```python
from build123d import *

# Parameters (mm, degrees)
SKETCH2_W                       = 1
SKETCH2_H                       = 27.5
REVOLVE1_ANGLE                  = 130
SKETCH3_W                       = 1
SKETCH3_H                       = 27.5
BOSS_EXTRUDE1_DEPTH             = 7.5
SKETCH4_W                       = 1
SKETCH4_H                       = 27.5
BOSS_EXTRUDE2_DEPTH             = 7.5
M2_5_CLEARANCE_HOLE1_D          = 3.1
CIRPATTERN1_COUNT               = 2
CIRPATTERN1_ANGLE               = 65
CIRPATTERN1_THE_OTHER_WAY_COUNT = 2
CIRPATTERN1_THE_OTHER_WAY_ANGLE = 65


with BuildPart() as part:
    # Sketch2 → Revolve1 (revolve, symmetric)
    with BuildSketch(Plane(origin=(0, 0, 0), x_dir=(0, 0, -1), z_dir=(1, 0, 0))) as revolve1_sk:
        with Locations((-149.5, 0)):
            Rectangle(SKETCH2_W, SKETCH2_H)
    revolve(axis=Axis((0, -1000, 0), (0, 1, 0)), revolution_arc=REVOLVE1_ANGLE / 2)
    revolve(revolve1_sk.sketch, axis=Axis((0, -1000, 0), (0, -1, 0)), revolution_arc=REVOLVE1_ANGLE / 2)

    # Sketch3 → Boss-Extrude1 (add)
    with BuildSketch(Plane(origin=(0, 0, 0), x_dir=(-0.9063077870366509, 1.4496858692468702e-15, -0.4226182617406975), z_dir=(0.4226182617406975, 3.1088613791648487e-15, -0.9063077870366509))):
        with Locations((-149.5, 0)):
            Rectangle(SKETCH3_W, SKETCH3_H)
    extrude(amount=BOSS_EXTRUDE1_DEPTH)

    # Sketch4 → Boss-Extrude2 (add)
    with BuildSketch(Plane(origin=(0, 0, 0), x_dir=(-0.906307787036651, -1.4496858692468694e-15, 0.4226182617406973), z_dir=(-0.4226182617406973, 3.1088613791648455e-15, -0.906307787036651))):
        with Locations((149.5, 0)):
            Rectangle(SKETCH4_W, SKETCH4_H)
    extrude(amount=BOSS_EXTRUDE2_DEPTH)

    # M2.5 Clearance Hole1 (through all)
    with Locations(Plane(origin=(0, 0, 0), x_dir=(1, 0, 0), z_dir=(0, 0, -1))):
        with Locations((0, -10.575), (0, 10.575)):
            m2_5_clearance_hole1 = Hole(M2_5_CLEARANCE_HOLE1_D / 2)

    # CirPattern1: M2.5 Clearance Hole1 ×2 about axis
    cirpattern1_axis = Axis((0, -1000, 0), (0, 1, 0))
    for i in range(1, CIRPATTERN1_COUNT):
        add(m2_5_clearance_hole1.rotate(cirpattern1_axis, i * CIRPATTERN1_ANGLE / (CIRPATTERN1_COUNT - 1)), mode=Mode.SUBTRACT)

    # CirPattern1 the other way: M2.5 Clearance Hole1 ×2 about axis
    cirpattern1_the_other_way_axis = Axis((0, -1000, 0), (0, -1, 0))
    for i in range(1, CIRPATTERN1_THE_OTHER_WAY_COUNT):
        add(m2_5_clearance_hole1.rotate(cirpattern1_the_other_way_axis, i * CIRPATTERN1_THE_OTHER_WAY_ANGLE / (CIRPATTERN1_THE_OTHER_WAY_COUNT - 1)), mode=Mode.SUBTRACT)


solid = part.part
```
For this review, take the finished solid that the model builds, in its own axes (mm). A direction names the side the tool comes from. Give positions to 0.01 mm unless a question says otherwise; leave off trailing zeros. Loops run counter-clockwise (first coordinate to the right, second up) from the corner with the lowest first, then second, coordinate; pieces in that order, holes last. Notation, with made-up numbers: M 21,17.5 L 75,17.5 A34 ccw 75,55.5 Z; hole C -21,7 d5. An arc over 180 degrees is marked long. One line per item, written item: value. Start each with the question number.
Q1. Add section D-D (x = 108). Give the boundary of the cut face in (y, z).
Q2. Add section C-C (x = -25). Give the boundary of the cut face in (y, z), and give its area (3 significant figures).
Q3. For L1, parallel to X at y = -11.5, z = 132.5; L2, parallel to X at y = 0, z = 98.5; L3, parallel to Z at x = -2, y = -10.75, list the stretches that pass through material, from the lowest coordinate up.
Q4. Add section A-A (z = 93.5). Give the boundary of the cut face in (x, y), and give its area (3 significant figures).
Q5. Machinability: for faces 1 (the face through (2.38, 0.19, 149.98)), 2 (the face through (-136.6, -0.19, 59.62)), which of the approach directions +Z, -Z, +X, -X, +Y, -Y give a long, thin tool a straight path to every point of the face, cutting with its end or side? Answer none if there is none.
Q6. Clearance check with flat-ended pins moving along their axes: pin 1 Ø2 at (x, y) = (-44.5, -6.5) entering from +Z; pin 2 Ø5 at (x, y) = (-71.5, 1.5) entering from -Z; pin 3 Ø10 at (y, z) = (5.5, 126.5) entering from -X. State where each tip first meets the part, or that it passes through.
Q7. Add section B-B (y = 5.75). Give the boundary of the cut face in (x, z), and give its area (3 significant figures).
Q8. Draft analysis for pull direction X (two halves, no side actions). For faces 3 (the face through (137.51, -0.19, 60.04)), 4 (the face through (-137.51, -0.19, 60.04)), 5 (the face through (136.6, -0.19, 59.62)), state which applies: released by +X, released by -X, zero draft, split by the parting line, or undercut.
Reply:
1. outline: M -13.75,102.65 L 13.75,102.65 L 13.75,104.1 L -13.75,104.1 Z
2. outline: M -13.75,146.89 L 13.75,146.89 L 13.75,147.9 L -13.75,147.9 Z
2. area: 27.9 mm²
3. L1: -70.31 to -68.15, 68.15 to 70.31
3. L2: -113.13 to -111.8, 111.8 to 113.13
3. L3: 148.99 to 149.99
4. outline: M -117.29,-13.75 L -116.01,-13.75 L -116.01,13.75 L -117.29,13.75 Z; M 116.01,-13.75 L 117.29,-13.75 L 117.29,13.75 L 116.01,13.75 Z
4. area: 70.5 mm²
5. face 1: +Z, +Y, -Y
5. face 2: -Z, +Y, -Y
6. pin 1: z = 143.55
6. pin 2: z = 129.33
6. pin 3: x = -87.96
7. outline: M -139.12,56.6 L -138.21,56.17 L -135.04,62.97 A149 cw 135.04,62.97 L 138.21,56.17 L 139.12,56.6 L 135.95,63.39 A150 ccw -135.95,63.39 Z
7. area: 354 mm²
8. face 3: released by +X
8. face 4: released by -X
8. face 5: undercut
